Input: part model. Units: mm. Frame: model coordinates. Face numbers are marked on the shaded views. A direction names the side the tool comes from. Coordinates: 2 decimals unless noted, no trailing zeros. Write each loop counter-clockwise with the first axis right and the second up, starting at its lowest first coordinate (ties: lowest second). Pieces come first, ordered by that corner, then holes. Notation, with made-up numbers: M -39.5,-31.5 L -31.5,-31.5 A32 cw -31.5,3.5 Z; hole C 22,64.25 d8. An arc over 180 degrees is marked long. Write each question's results on one line, items separated by ' | '. Start each with the question number.
1. Section query A-A, the plane x = 167. Output: boundary loops of the cut face in (y, z), and give its area (3 significant figures).
2. Ray query, probe 1 along Z at (x, y) = (106.5, -13); probe 2 along Y at (x, z) = (30, 9.6); probe 3 along Y at (x, z) = (30, 11.3). Return the intervals inside material, ascending.
3. Set-up query: the marked faces 1 and 2. Return all of +Z, -Z, +X, -X, +Y, -Y with unobstructed straight access to the full face (end or side cutting, diameter ignored); none if empty.
4. First-contact query: pin 1 (4 mm diameter, centred on y = -15.5, z = 10.5, fed in from -X); pin 2 (12 mm diameter, centred on x = 173, y = 9.5, fed in from +Z); pin 3 (1.5 mm diameter, centred on x = 131, z = 11, fed in from -Y); pin 4 (2.5 mm diameter, centred on x = 30, y = -6.9, fed in from +Z). Flat tips, straight axial feed; report the tip coordinate or a pass-through.
5. Section query B-B, the plane y = -12.5. Output: boundary loops of the cut face in (x, z).
Autodesk Inventor part; units mm, degrees
ref_plane "YZ Plane" through (0, 0, 0) normal (1, 0, 0) x (0, 1, 0)
ref_plane "XZ Plane" through (0, 0, 0) normal (0, 1, 0) x (-1, 0, 0)
ref_plane "XY Plane" through (0, 0, 0) normal (0, 0, 1) x (1, 0, 0)
sketch "Sketch1" plane through (0, 0, 0) normal (1, 0, 0) x (0, 1, 0)
  circle A0 centre (0, 0) radius 20
  line L0 (8.5, 8.5) -> (-16.9, 8.5)
  line L1 (8.5, 8.5) -> (8.5, -16.9)
  line L2 (0, 0) -> (0, 20)
  line L3 (0, 20) -> (-60.9241, 20)
  line L4 (-60.9241, 20) -> (-60.9241, 18.5)
  line L5 (-60.9241, 18.5) -> (0, 18.5)
  line L6 (0, 18.5) -> (0, 20)
  line L7 (0, 0) -> (14.1421, 14.1421)
  line L8 (0, 0) -> (20, 0)
  line L9 (-16.9, 8.5) -> (-16.9, 18.5)
  line L10 (-16.9, 8.5) -> (-22.9, 14.5)
  line L11 (-22.9, 14.5) -> (-22.9, 18.5)
  line L12 (12.3744, 12.3744) -> (12.1502, 13.2109)
  line L13 (11.3137, 13.435) -> (9.2071, 11.3284)
  line L14 (9.4313, 10.4919) -> (10.2678, 10.2678)
  line L15 (8.5, 8.5) -> (8.5, -16.9)
  line L16 (20, 0) -> (20, -60.9241)
  line L17 (20, -60.9241) -> (18.5, -60.9241)
  line L18 (18.5, -60.9241) -> (18.5, 0)
  line L19 (8.5, -16.9) -> (18.5, -16.9)
  line L20 (8.5, -16.9) -> (14.5, -22.9)
  line L21 (14.5, -22.9) -> (18.5, -22.9)
  arc A1 (9.2071, 11.3284) -> (9.4313, 10.4919) centre (9.5607, 10.9749) ccw
  arc A2 (12.1502, 13.2109) -> (11.3137, 13.435) centre (11.6673, 13.0815) ccw
  line L22 (10.4311, 10.4311) -> (9.483, 10.6851)
  arc A3 (9.3485, 11.187) -> (9.483, 10.6851) centre (9.5607, 10.9749) ccw
  line L23 (9.3485, 11.187) -> (11.4551, 13.2936)
  arc A4 (11.957, 13.1591) -> (11.4551, 13.2936) centre (11.6673, 13.0815) ccw
  line L24 (11.957, 13.1591) -> (12.2111, 12.2111)
  point P0 (0, 8.5)
  point P1 (-17.7041, 9.3041)
  point P2 (-16.9, 10.6953)
  dimension "d0" = 40
  dimension "d1" = 25.4
  dimension "d2" = 1.5
  dimension "d4" = 45
  dimension "d6" = 45
  dimension "d7" = 4
  dimension "d8" = 10
  dimension "d10" = 2.5
  dimension "d11" = 2.5
  dimension "d12" = 60
  dimension "d13" = 1.5
  dimension "d15" = 0.5
  dimension "d16" = 0.2
extrude "Extrusion1" add sketch "Sketch1" along normal blind 216 contours L7 L12 A2 L13 A1 L14 L0 L2 A0 | L7 L24 A4 L23 A3 L22 L14 A1 L13 A2 L12 | L5 L2 L0 L9 A0 | A0 L9 L5 | L7 L22 A3 L23 A4 L24 | L9 L10 A0 | A0 L10 L11 L5 L9
sketch "Sketch2" plane through (0, -22.9, 18.5) normal (0, 0, 1) x (1, 0, 0)
  line L0 (0, 22.9) -> (0, 0)
  line L1 (0, 0) -> (216, 0)
  line L2 (216, 22.9) -> (216, 0)
  line L3 (0, 22.9) -> (216, 22.9)
  line L4 (28.3257, 13.1) -> (26.6514, 16)
  line L5 (26.6514, 16) -> (28.3257, 18.9)
  line L6 (28.3257, 18.9) -> (31.6743, 18.9)
  line L7 (31.6743, 18.9) -> (33.3486, 16)
  line L8 (33.3486, 16) -> (31.6743, 13.1)
  line L9 (31.6743, 13.1) -> (28.3257, 13.1)
  line L10 (0, 6) -> (216, 6)
  circle A0 centre (30, 16) radius 1.65
  dimension "d20" = 10
  dimension "d21" = 5.8
  dimension "d22" = 30
  dimension "d25" = 3.3
extrude "Extrusion2" cut sketch "Sketch2" against normal blind 6 contours L4 L5 L6 L7 L8 L9 | A0
extrude "Extrusion3" cut sketch "Sketch2" against normal through all contours A0
sketch "Sketch3" plane through (0, -22.9, 18.5) normal (0, 0, 1) x (1, 0, 0)
  line L0 (0, 37.0421) -> (216, 37.0421)
  line L1 (0, 0) -> (216, 0)
  line L2 (0, 22.9) -> (0, 0)
  line L3 (0, 22.9) -> (0, 37.0421)
  line L4 (2.4384, 37.0421) -> (17.8575, 0)
  line L5 (0, 0) -> (216, 0)
  line L6 (2.4384, 37.0421) -> (0, 42.9)
  point P0 (0, 26.9698)
  dimension "d28" = 112.6
sketch "Sketch4" plane through (216, 14.1421, 14.1421) normal (0, 0.7071, -0.7071) x (-1, 0, 0)
  line L0 (216, 0) -> (0, 0)
  line L1 (0, -7.9792) -> (0, 0)
  line L2 (216, -7.9792) -> (0, -7.9792)
  circle A0 centre (20, -4) radius 1.5
  circle A1 centre (110, -4) radius 1.5
  circle A2 centre (200, -4) radius 1.5
  line L3 (216, -7.9792) -> (216, 0)
  point P0 (216, -20)
  dimension "d34" = 3
  dimension "d35" = 4
  dimension "d36" = 20
  dimension "d39" = 90
extrude "Extrusion5" cut sketch "Sketch4" against normal blind 3 contours A0 | A1 | A2
extrude "Extrusion6" cut sketch "Sketch3" along normal through all both and the other way through all
properties part number "ESQUINA_REDONDEADA_R20" material "Steel, Mild, Welded"
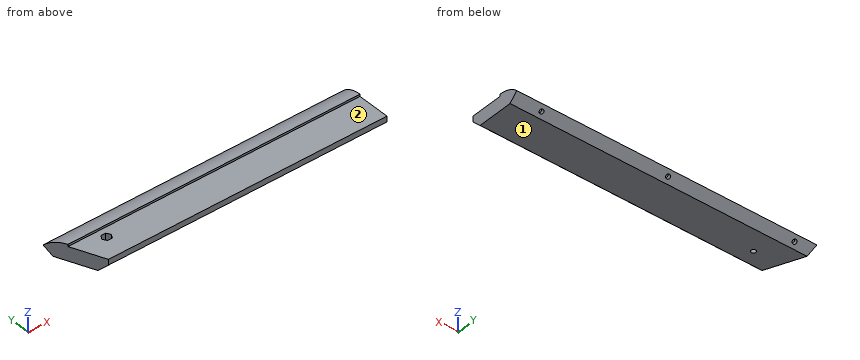
Answer:
1) outline: M -22.9,14.5 L -16.9,8.5 L 8.5,8.5 L 14.14,14.14 A20 ccw 0,20 L 0,18.5 L -22.9,18.5 Z | area: 332 mm^2
2) probe 1: 8.5 to 18.5 | probe 2: -18 to -8.55, -5.25 to 9.6 | probe 3: -19.7 to -8.55, -5.25 to 11.3
3) face 1: -Z, +X, -X, +Y, -Y | face 2: +Z, +X, -X, -Y
4) pin 1: x = 13.94 | pin 2: z = 19.69 | pin 3: y = -20.15 | pin 4: through
5) outline: M 13.53,8.5 L 216,8.5 L 216,18.5 L 13.53,18.5 Z
